from build123d import *

# Parameters (mm, degrees)
SKETCH1_R                       = 50.165
BOSS_EXTRUDE1_DEPTH             = 20.32
SKETCH4_W                       = 6.858
SKETCH4_H                       = 39.37
BOSS_EXTRUDE3_DEPTH             = 7.62
BOSS_EXTRUDE4_DEPTH             = 31.242
BOSS_EXTRUDE5_DEPTH             = 15.24
F_4_0MM_DOWEL_HOLE1_D           = 4
F_4_0MM_DOWEL_HOLE1_DEPTH       = 3.81
F_4_0MM_DOWEL_HOLE1_CSINK_D     = 4.05
F_4_0MM_DOWEL_HOLE1_CSINK_ANGLE = 100
F_4_0MM_DOWEL_HOLE1_TIP         = 1.201721238
F_4_0MM_DOWEL_HOLE2_D           = 4
F_4_0MM_DOWEL_HOLE2_DEPTH       = 3.81
F_4_0MM_DOWEL_HOLE2_CSINK_D     = 4.05
F_4_0MM_DOWEL_HOLE2_CSINK_ANGLE = 100
F_4_0MM_DOWEL_HOLE2_TIP         = 1.201721238


with BuildPart() as part:
    # Sketch1 → Boss-Extrude1 (new body)
    with BuildSketch(Plane.XY):
        Circle(SKETCH1_R)
        with BuildLine():
            Line((16.764, -19.685), (23.622, -19.685))
            Line((23.622, -19.685), (23.622, 19.685))
            Line((23.622, 19.685), (-23.622, 19.685))
            Line((-23.622, 19.685), (-23.622, -19.685))
            Line((-23.622, -19.685), (-16.764, -19.685))
            ThreePointArc((-16.764, -19.685), (0, -29.98053413), (16.764, -19.685))
        make_face(mode=Mode.SUBTRACT)
    extrude(amount=BOSS_EXTRUDE1_DEPTH)

    # Sketch4 → Boss-Extrude3 (add)
    with BuildSketch(Plane(origin=(0, 0, 0), x_dir=(-1, 0, 0), z_dir=(0, 0, -1))):
        with Locations((-20.193, 0)):
            Rectangle(SKETCH4_W, SKETCH4_H)
        with Locations((20.193, 0)):
            Rectangle(SKETCH4_W, SKETCH4_H)
    extrude(amount=-BOSS_EXTRUDE3_DEPTH)

    # Sketch5 → Boss-Extrude4 (add)
    with BuildSketch(Plane.XY.offset(20.32)):
        with BuildLine():
            ThreePointArc((-18.288, -21.463), (0, -31.496), (18.288, -21.463))
            Line((18.288, -21.463), (25.4, -21.463))
            Line((25.4, -21.463), (25.4, 21.463))
            Line((25.4, 21.463), (-25.4, 21.463))
            Line((-25.4, 21.463), (-25.4, -21.463))
            Line((-25.4, -21.463), (-18.288, -21.463))
        make_face()
        with BuildLine():
            Line((-16.764, -19.685), (-23.622, -19.685))
            Line((-23.622, -19.685), (-23.622, 19.685))
            Line((-23.622, 19.685), (23.622, 19.685))
            Line((23.622, 19.685), (23.622, -19.685))
            Line((23.622, -19.685), (16.764, -19.685))
            ThreePointArc((16.764, -19.685), (0, -29.98053413), (-16.764, -19.685))
        make_face(mode=Mode.SUBTRACT)
    extrude(amount=BOSS_EXTRUDE4_DEPTH)

    # Sketch6 → Boss-Extrude5 (add)
    with BuildSketch(Plane.XY.offset(20.32)):
        with BuildLine():
            Line((13.809066775, -48.226931271), (13.49453303, -45.962673219))
            ThreePointArc((13.49453303, -45.962673219), (0.162084285, -47.884773517), (-13.179792846, -46.029248327))
            Line((-13.179792846, -46.029248327), (-13.809066775, -48.226931271))
            ThreePointArc((-13.809066775, -48.226931271), (0, -50.165), (13.809066775, -48.226931271))
        make_face()
        with BuildLine():
            Line((-12.94251142, 48.466675388), (-12.507062463, 46.222531853))
            ThreePointArc((-12.507062463, 46.222531853), (0.054767522, 48.038227874), (12.611793827, 46.189602713))
            Line((12.611793827, 46.189602713), (13.293700106, 48.371528428))
            ThreePointArc((13.293700106, 48.371528428), (0.181924735, 50.164670121), (-12.94251142, 48.466675388))
        make_face()
    extrude(amount=BOSS_EXTRUDE5_DEPTH)

    # Ø4.0mm Dowel Hole1
    with Locations(Plane(origin=(-0.291325712, 50.164154078, 27.945133858), x_dir=(0.999983137201, 0.005807349979, 0), z_dir=(-0.005807349979, 0.999983137201, 0))):
        with Locations((0, 0)):
            CounterSinkHole(F_4_0MM_DOWEL_HOLE1_D / 2, F_4_0MM_DOWEL_HOLE1_CSINK_D / 2, depth=F_4_0MM_DOWEL_HOLE1_DEPTH, counter_sink_angle=F_4_0MM_DOWEL_HOLE1_CSINK_ANGLE)
            with Locations((0, 0, -(F_4_0MM_DOWEL_HOLE1_DEPTH + F_4_0MM_DOWEL_HOLE1_TIP / 2))):  # 118° drill point
                Cone(0, F_4_0MM_DOWEL_HOLE1_D / 2, F_4_0MM_DOWEL_HOLE1_TIP, mode=Mode.SUBTRACT)

    # Ø4.0mm Dowel Hole2
    with Locations(Plane(origin=(-0.253466909, -50.164359654, 27.907450527), x_dir=(-0.99998723521, 0.005052664379, 0), z_dir=(-0.005052664379, -0.99998723521, 0))):
        with Locations((0, 0)):
            CounterSinkHole(F_4_0MM_DOWEL_HOLE2_D / 2, F_4_0MM_DOWEL_HOLE2_CSINK_D / 2, depth=F_4_0MM_DOWEL_HOLE2_DEPTH, counter_sink_angle=F_4_0MM_DOWEL_HOLE2_CSINK_ANGLE)
            with Locations((0, 0, -(F_4_0MM_DOWEL_HOLE2_DEPTH + F_4_0MM_DOWEL_HOLE2_TIP / 2))):  # 118° drill point
                Cone(0, F_4_0MM_DOWEL_HOLE2_D / 2, F_4_0MM_DOWEL_HOLE2_TIP, mode=Mode.SUBTRACT)


solid = part.part
Can you work these out from the model? Positions are in its coordinate system, mm. A direction names the side the tool comes from. Coordinates: 2 decimals unless noted, no trailing zeros. Order: outer loops, then holes, each group sorted by start corner. A loop starts at its lowest first (then second) coordinate and runs counter-clockwise, first axis right, second up. Notation, with made-up numbers: M 21,56.5 L 77,56.5 A28 cw 77,88.5 Z; hole C 88.25,85.25 d2. An arc over 180 degrees is marked long. Write item = value, one per line.
(1) I need wall thicknesses on line 1 along X through (y, z) = (0, 47); line 2 along Y through (x, z) = (19, 38.5) (3 decimals); line 3 along Z through (x, y) = (21, 36). Which ranges of each line are inside material? Lowest first, please. Write a range as [from, to].
Results are:
line_1 = [-25.4, -23.62], [23.62, 25.4]
line_2 = [-21.463, -19.685], [19.685, 21.463]
line_3 = [0, 20.32]
(2) Suppose I cut it at A-A on y = 0. Please give me the cut outline in (x, z) (3 decimals), plus the area to 3 significant figures.
Results are:
outline = M -50.165,0 L -16.764,0 L -16.764,7.62 L -23.622,7.62 L -23.622,51.562 L -25.4,51.562 L -25.4,20.32 L -50.165,20.32 Z; M 16.764,0 L 50.165,0 L 50.165,20.32 L 25.4,20.32 L 25.4,51.562 L 23.622,51.562 L 23.622,7.62 L 16.764,7.62 Z
area = 1,290 mm2
(3) Suppose I cut it at D-D on z = 19. Please give me the cut outline in (x, y) (3 decimals), plus the area to 3 significant figures.
Results are:
outline = C 0,0 d100.33; hole M -23.622,-19.685 L -16.764,-19.685 A18.796 ccw 16.764,-19.685 L 23.622,-19.685 L 23.622,19.685 L -23.622,19.685 Z
area = 5,800 mm2
(4) Suppose I cut it at C-C on x = 5.5. Please give me the cut outline in (y, z) (3 decimals), plus the area to 3 significant figures.
Results are:
outline = M -49.863,0 L -29.158,0 L -29.158,51.562 L -30.787,51.562 L -30.787,20.32 L -47.574,20.32 L -47.574,35.56 L -49.863,35.56 Z; M 19.685,0 L 49.863,0 L 49.863,35.56 L 47.693,35.56 L 47.693,20.32 L 21.463,20.32 L 21.463,51.562 L 19.685,51.562 Z
area = 1,210 mm2
(5) For pin 1 Ø14 at (x, z) = (11.5, 23) entering from -Y; pin 2 Ø5 at (y, z) = (31, 10.5) entering from -X; pin 3 Ø2 at (x, y) = (4.5, 49) entering from +Z, each with a flat end and sliding along its axis, tell me the tip position at first contact or that it passes through.
Results are:
pin_1 = -49.96
pin_2 = -41.28
pin_3 = 35.56
(6) If we mould it in two halves opening along Y, with no side actions, what happens to faces 1 (the face through (-22, -21.463, 36)), 2 (the face through (-2.95, 47.94, 27.83)), 3 (the face through (25.4, 0, 36)), 4 (the face through (-23.622, 0, 29))? For each: pulls with the +Y half, pulls with the -Y half, needs draft (parallel to the pull), parting line crosses it, or undercut.
Results are:
face_1 = pulls with the -Y half
face_2 = undercut
face_3 = needs draft
face_4 = undercut
(7) Suppose I cut it at B-B on z = 43.5. Please give me the cut outline in (x, y) (3 decimals).
Results are:
outline = M -25.4,-21.463 L -18.288,-21.463 A21.684 ccw 18.288,-21.463 L 25.4,-21.463 L 25.4,21.463 L -25.4,21.463 Z; hole M -23.622,-19.685 L -16.764,-19.685 A18.796 ccw 16.764,-19.685 L 23.622,-19.685 L 23.622,19.685 L -23.622,19.685 Z
(8) For faces 5 (the face through (0, 21.463, 36)), 6 (the face through (-25.4, 0, 36)), 7 (the face through (-20, -19.685, 29)), 8 (the face through (16.764, 0, 4)), which set-ups out of +Z, -Z, +X, -X, +Y, -Y let a thin tool reach every point of the face, with its end or its side?
Results are:
face_5 = +Z, +X, -X
face_6 = +Z, -X, +Y, -Y
face_7 = +Z
face_8 = +Z, -Z
